The listing builds one solid part. Answer for the finished solid, in the listing's coordinates (mm). Coordinates: 2 decimals unless noted, no trailing zeros. Write each loop counter-clockwise with the first axis right and the second up, starting at its lowest first coordinate (ties: lowest second). Pieces come first, ordered by that corner, then holes.
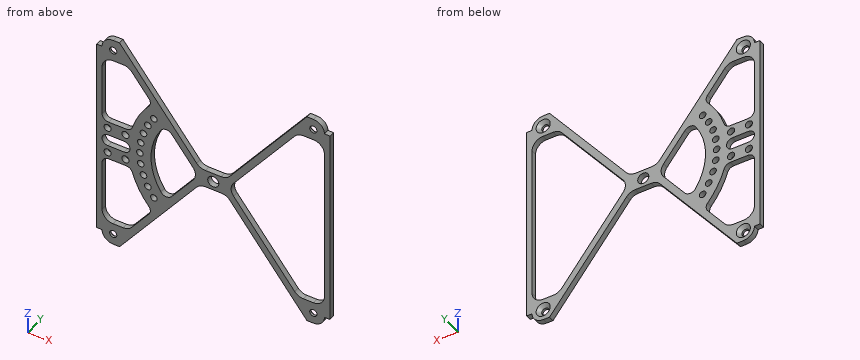
from build123d import *

# Parameters (mm, degrees)
SKETCH1_R           = 1.625
SKETCH1_R_2         = 2.5
BOSS_EXTRUDE1_DEPTH = 2.5
FILLET1_R           = 5
FILLET2_R           = 5
CHAMFER1_SIZE       = 1.55
SKETCH3_R           = 1.625
SKETCH3_R_2         = 1.5
BOSS_EXTRUDE2_DEPTH = 2.5
FILLET3_R           = 3


with BuildPart() as part:
    # Sketch1 → Boss-Extrude1 (new body)
    with BuildSketch(Plane(origin=(0, 0, 0), x_dir=(1, 0, 0), z_dir=(0, 1, 0))):
        with BuildLine():
            Line((-52.5, 45), (-52.5, -45))
            Line((-52.5, -45), (-50, -45))
            ThreePointArc((-50, -45), (-48.535533906, -48.535533906), (-45, -50))
            Line((-45, -50), (-42.127158908, -50))
            Line((-42.127158908, -50), (-6, -4))
            Line((-6, -4), (6, -4))
            Line((6, -4), (42.127158908, -50))
            Line((42.127158908, -50), (45, -50))
            ThreePointArc((45, -50), (48.535533906, -48.535533906), (50, -45))
            Line((50, -45), (52.5, -45))
            Line((52.5, -45), (52.5, 45))
            Line((52.5, 45), (50, 45))
            ThreePointArc((50, 45), (48.535533906, 48.535533906), (45, 50))
            Line((45, 50), (42.127158908, 50))
            Line((42.127158908, 50), (6, 4))
            Line((6, 4), (-6, 4))
            Line((-6, 4), (-42.127158908, 50))
            Line((-42.127158908, 50), (-45, 50))
            ThreePointArc((-45, 50), (-48.535533906, 48.535533906), (-50, 45))
            Line((-50, 45), (-52.5, 45))
        make_face()
        with Locations(Location((-45, 45, 0), (0, 0, 270))):
            Circle(SKETCH1_R, mode=Mode.SUBTRACT)
        with Locations(Location((45, 45, 0), (0, 0, 270))):
            Circle(SKETCH1_R, mode=Mode.SUBTRACT)
        with Locations(Location((-45, -45, 0), (0, 0, 270))):
            Circle(SKETCH1_R, mode=Mode.SUBTRACT)
        with Locations(Location((45, -45, 0), (0, 0, 270))):
            Circle(SKETCH1_R, mode=Mode.SUBTRACT)
        with Locations(Location((0, 0, 0), (0, 0, 270))):
            Circle(SKETCH1_R_2, mode=Mode.SUBTRACT)
        Polygon((-50, 40), (-50, -40), (-38.088044946, -40), (-6.673124156, 0), (-38.088044946, 40), align=None, mode=Mode.SUBTRACT)
        Polygon((50, -40), (38.088044946, -40), (6.673124156, 0), (38.088044946, 40), (50, 40), align=None, mode=Mode.SUBTRACT)
    extrude(amount=BOSS_EXTRUDE1_DEPTH)

    # Fillet1
    fillet1_edges = [part.edges().sort_by_distance(p)[0] for p in [
        (-6, 1.25, -4),
        (6, 1.25, -4),
        (6, 1.25, 4),
        (-6, 1.25, 4),
        (-6.673124156, 1.25, 0),
        (6.673124156, 1.25, 0),
    ]]
    fillet(fillet1_edges, radius=FILLET1_R)

    # Fillet2
    fillet2_edges = [part.edges().sort_by_distance(p)[0] for p in [
        (-38.088044946, 1.25, -40),
        (-50, 1.25, -40),
        (-50, 1.25, 40),
        (-38.088044946, 1.25, 40),
        (50, 1.25, 40),
        (50, 1.25, -40),
        (38.088044946, 1.25, -40),
        (38.088044946, 1.25, 40),
    ]]
    fillet(fillet2_edges, radius=FILLET2_R)

    # Chamfer1
    chamfer1_edges = [part.edges().sort_by_distance(p)[0] for p in [
        (-45, 2.5, -46.625),
        (45, 2.5, -46.625),
        (-45, 2.5, 43.375),
        (45, 2.5, 43.375),
    ]]
    chamfer(chamfer1_edges, length=CHAMFER1_SIZE)

    # Sketch3 → Boss-Extrude2 (add)
    with BuildSketch(Plane(origin=(0, 2.5, 0), x_dir=(1, 0, 0), z_dir=(0, 1, 0))):
        with BuildLine():
            Line((-27.373335632, 26.357171631), (-21.115199634, 18.388810304))
            ThreePointArc((-21.115199634, 18.388810304), (-28, 0), (-21.115199634, -18.388810304))
            Line((-21.115199634, -18.388810304), (-27.373335632, -26.357171631))
            ThreePointArc((-27.373335632, -26.357171631), (-33.296974163, -18.311513088), (-36.918829884, -9))
            Line((-36.918829884, -9), (-52.5, -9))
            Line((-52.5, -9), (-52.5, 9))
            Line((-52.5, 9), (-36.918829884, 9))
            ThreePointArc((-36.918829884, 9), (-33.296974163, 18.311513088), (-27.373335632, 26.357171631))
        make_face()
        with Locations(Location((-47.5, 6, 0), (0, 0, 270))):
            Circle(SKETCH3_R, mode=Mode.SUBTRACT)
        with Locations(Location((-39.5, 6, 0), (0, 0, 270))):
            Circle(SKETCH3_R, mode=Mode.SUBTRACT)
        with Locations(Location((-39.5, -6, 0), (0, 0, 90))):
            Circle(SKETCH3_R, mode=Mode.SUBTRACT)
        with Locations(Location((-47.5, -6, 0), (0, 0, 90))):
            Circle(SKETCH3_R, mode=Mode.SUBTRACT)
        with Locations(Location((-33, 0, 0), (0, 0, 270))):
            Circle(SKETCH3_R_2, mode=Mode.SUBTRACT)
        with Locations(Location((-32.59371524, 5.162337346, 0), (0, 0, 270))):
            Circle(SKETCH3_R_2, mode=Mode.SUBTRACT)
        with Locations(Location((-31.384865038, 10.197560814, 0), (0, 0, 270))):
            Circle(SKETCH3_R_2, mode=Mode.SUBTRACT)
        with Locations(Location((-29.403215298, 14.981686491, 0), (0, 0, 270))):
            Circle(SKETCH3_R_2, mode=Mode.SUBTRACT)
        with Locations(Location((-26.697560814, 19.396913326, 0), (0, 0, 270))):
            Circle(SKETCH3_R_2, mode=Mode.SUBTRACT)
        with Locations(Location((-26.697560814, -19.396913326, 0), (0, 0, 270))):
            Circle(SKETCH3_R_2, mode=Mode.SUBTRACT)
        with Locations(Location((-29.403215298, -14.981686491, 0), (0, 0, 270))):
            Circle(SKETCH3_R_2, mode=Mode.SUBTRACT)
        with Locations(Location((-31.384865038, -10.197560814, 0), (0, 0, 270))):
            Circle(SKETCH3_R_2, mode=Mode.SUBTRACT)
        with Locations(Location((-32.59371524, -5.162337346, 0), (0, 0, 270))):
            Circle(SKETCH3_R_2, mode=Mode.SUBTRACT)
        with BuildLine():
            Line((-47.353810883, 2.646189117), (-40.079768039, 2.646189117))
            ThreePointArc((-40.079768039, 2.646189117), (-37.433578922, 0), (-40.079768039, -2.646189117))
            Line((-40.079768039, -2.646189117), (-47.353810883, -2.646189117))
            ThreePointArc((-47.353810883, -2.646189117), (-50, 0), (-47.353810883, 2.646189117))
        make_face(mode=Mode.SUBTRACT)
    extrude(amount=-BOSS_EXTRUDE2_DEPTH)

    # Fillet3
    fillet3_edges = [part.edges().sort_by_distance(p)[0] for p in [
        (-50, 1.25, -9),
        (-50, 1.25, 9),
        (-36.918829884, 1.25, -9),
        (-27.373335632, 1.25, -26.357171631),
        (-21.115199634, 1.25, -18.388810304),
        (-21.115199634, 1.25, 18.388810304),
        (-27.373335632, 1.25, 26.357171631),
        (-36.918829884, 1.25, 9),
    ]]
    fillet(fillet3_edges, radius=FILLET3_R)


solid = part.part
Q1. The part is cut by section C-C, the plane y = 1.4. State how many separate pieces and enclosed holes the cut face has, then the cut area to 3 significant figures.
Answers below:
separate pieces: 1
enclosed holes: 23
area: 2,110 mm2
Q2. The part is cut by section A-A, the plane z = 0. Write down the section's boundary in (x, y).
Answers below:
outline: (-52.5, 0) - (-50, 0) - (-50, 2.5) - (-52.5, 2.5) - close; (-37.43, 0) - (-34.5, 0) - (-34.5, 2.5) - (-37.43, 2.5) - close; (-31.5, 0) - (-28, 0) - (-28, 2.5) - (-31.5, 2.5) - close; (-8.03, 0) - (-2.5, 0) - (-2.5, 2.5) - (-8.03, 2.5) - close; (2.5, 0) - (8.03, 0) - (8.03, 2.5) - (2.5, 2.5) - close; (50, 0) - (52.5, 0) - (52.5, 2.5) - (50, 2.5) - close
Q3. Find the intervals of material crossed by probe 1 along Z at (x, y) = (2, 0.1); probe 2 along X at (y, z) = (0.35, 28.5); probe 3 along Z at (x, y) = (-37, 0.3), in increasing order.
Answers below:
probe 1: z = -4 to -1.5, 1.5 to 4
probe 2: x = -52.5 to -50, -29.06 to -25.24, 25.24 to 29.06, 50 to 52.5
probe 3: z = -43.47 to -38.55, -9.97 to 9.97, 38.55 to 43.47
Q4. Given pin 1 (0.8 mm diameter, centred on x = -52, y = 1.5, fed in from -Z); pin 2 (3 mm diameter, centred on x = -39.5, z = -6, fed in from +Y), each flat-ended and moving along its own axis, determine where each tip first touches the part or whether it passes through.
Answers below:
pin 1: stops at z = -45
pin 2: passes through
Q5. The part is cut by section B-B, the plane x = 33.5. Write down the section's boundary in (y, z).
Answers below:
outline: (0, -39.02) - (2.5, -39.02) - (2.5, -34.16) - (0, -34.16) - close; (0, 34.16) - (2.5, 34.16) - (2.5, 39.02) - (0, 39.02) - close
